Build history of the part. All positions in model axes, mm. A direction names the side the tool comes from. Give positions to 0.01 mm unless a question says otherwise; leave off trailing zeros. Order: outer loops, then holes, each group sorted by start corner. A loop starts at its lowest first (then second) coordinate and runs counter-clockwise, first axis right, second up. Notation, with made-up numbers: (-2, 57.25) -> (57, 57.25) arc R13 ccw to (57, 70.25) -> close; hole circle Ø6 at (38.5, -2.5). An arc over 180 degrees is marked (long way). One line per item, written item: value. Start each with the question number.
(1) Probe line 1 (Z direction, x = 8, y = 0); line 2 (X direction, y = 33, z = 55); line 3 (Y direction, x = 11, z = 10.5). List the from-to ranges inside material, lowest first.
(2) Which spindle directions (+Z, -Z, +X, -X, +Y, -Y) get a long thin tool onto all of the face, cutting with end or side? Do faces 4 (the cylindrical face through (7.957, -15.485, 69.733)), 5 (the flat face through (10.312, 30, 30)), 6 (the flat face through (-10.312, -30, 30)), 7 (the conical face through (-4.724, 29.706, 57.114)), 8 (the flat face through (16.669, 15, 15)). Say none if no direction does.
(3) Pin check, flat tips, straight feed: pin 1 (12 mm diameter, centred on y = 44, z = 25, fed in from +X); pin 2 (1 mm diameter, centred on x = 12, z = 8, fed in from -Y); pin 3 (1.5 mm diameter, centred on y = 38, z = -3.5, fed in from -X). Stop position of each tip, or through.
(4) Saw through at D-D on x = -2. Give the cut face in (y, z).
(5) Two-plate mould, pull along Z, no slides. Class faces 1 (the cylindrical face through (-7.912, -15.485, 69.733)), 2 (the flat face through (-16.669, -15, 15)), 3 (the cylindrical face through (0.233, -15.128, -11.599)): +Z half, -Z half, draft (parallel to the pull), parting line (faces both ways), or undercut.
(6) Saw through at C-C on x = -14. Give the cut face in (y, z), plus the area to 3 significant figures.
```python
from build123d import *

# Parameters (mm, degrees)
SKETCH2_R          = 19.0627
CUT_EXTRUDE1_DEPTH = 34.3375


with BuildPart() as part:
    # Sketch1 → Revolve1 (revolve)
    with BuildSketch(Plane.XY):
        with BuildLine():
            Line((16.66875, 0), (-16.66875, 0))
            Line((-16.66875, 0), (-16.66875, 34.891972302))
            Line((-16.66875, 34.891972302), (-16.6624, 34.891972302))
            ThreePointArc((-16.6624, 34.891972302), (-12.172271939, 36.751844242), (-10.3124, 41.241972302))
            Line((-10.3124, 41.241972302), (-10.3124, 70.6374))
            Line((-10.3124, 70.6374), (-9.51865, 71.43115))
            Line((-9.51865, 71.43115), (-6.35, 71.43115))
            Line((-6.35, 71.43115), (-4.640755559, 64.017549491))
            ThreePointArc((-4.640755559, 64.017549491), (0, 60.325), (4.640755559, 64.017549491))
            Line((4.640755559, 64.017549491), (6.35, 71.43115))
            Line((6.35, 71.43115), (9.51865, 71.43115))
            Line((9.51865, 71.43115), (10.3124, 70.6374))
            Line((10.3124, 70.6374), (10.3124, 41.241972302))
            ThreePointArc((10.3124, 41.241972302), (12.172271939, 36.751844242), (16.6624, 34.891972302))
            Line((16.6624, 34.891972302), (16.66875, 34.891972302))
            Line((16.66875, 34.891972302), (16.66875, 0))
        make_face()
    revolve(axis=Axis((16.66875, 0, 0), (-1, 0, 0)))

    # Sketch2 → Cut-Extrude1 (cut, through all)
    with BuildSketch(Plane(origin=(16.66875, 0, 0), x_dir=(0, 0, -1), z_dir=(1, 0, 0))):
        with Locations(Location((0, 0, 0), (0, 0, 90))):  # turned: the seam where the file's is
            Circle(SKETCH2_R)
    extrude(amount=-CUT_EXTRUDE1_DEPTH, mode=Mode.SUBTRACT)


solid = part.part
```
Results below:
1. line 1: z = -71.43 to -19.06, 19.06 to 71.43
1. line 2: x = -10.31 to -4.67, 4.67 to 10.31
1. line 3: y = -36.9 to -15.91, 15.91 to 36.9
2. face 4: +X, -X
2. face 5: +X
2. face 6: -X
2. face 7: none
2. face 8: +Z, -Z, +X, +Y, -Y
3. pin 1: stops at x = 10.31
3. pin 2: stops at y = -36.69
3. pin 3: stops at x = -11.6
4. outline: circle Ø121.53 at (0, 0); hole circle Ø38.13 at (0, 0)
5. face 1: parting line
5. face 2: draft
5. face 3: undercut
6. outline: circle Ø70.95 at (0, 0); hole circle Ø38.13 at (0, 0)
6. area: 2,810 mm²
